For this review, use the dimensioned drawing (mm, ordinates from the lowest corner) and the shaded views. A direction names the side the tool comes from. Round coordinates to 2 decimals unless told otherwise and drop trailing zeros. Write each loop counter-clockwise with the first axis right and the second up, starting at its lowest first coordinate (ties: lowest second). Pieces come first, ordered by that corner, then holes. Notation, with made-up numbers: M 39.5,52 L 55.5,52 A18 cw 55.5,65 Z; hole C -35.5,-16.75 d10. An arc over 180 degrees is marked long. Write each question's results on one line, items separated by ' | '. Start each with the question number.
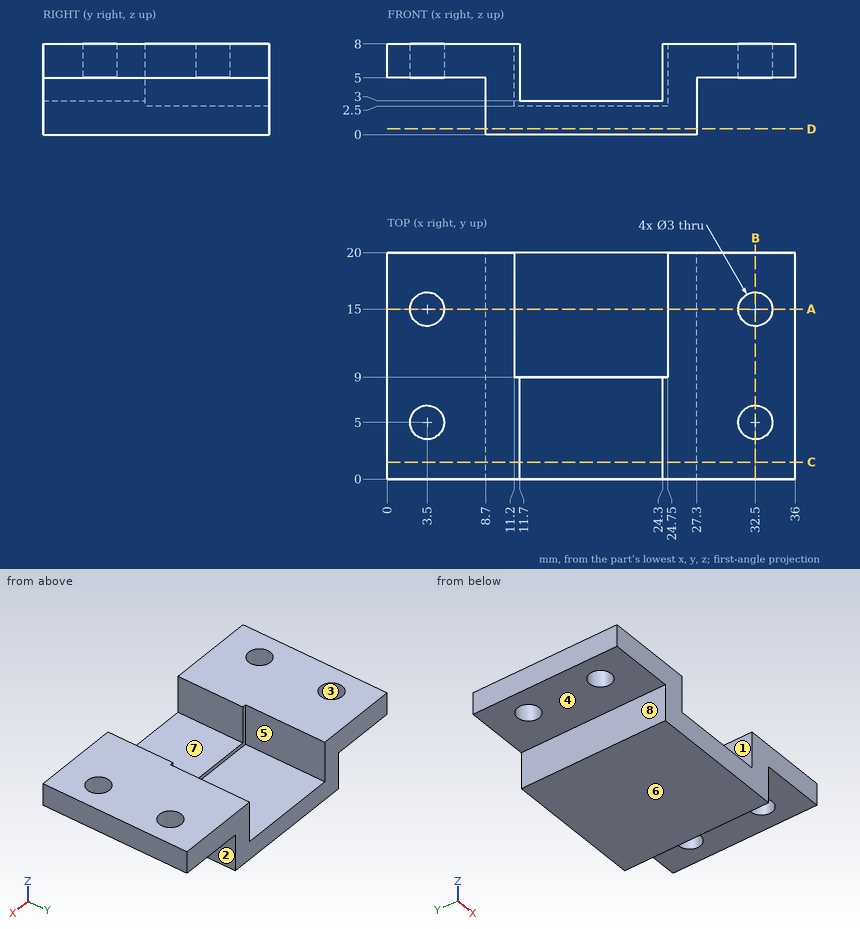
Item 1: Insertion check: P1, Ø3.5, axis at x = 15.5, y = 13, coming from the +Z side; P2, Ø7, axis at x = 19.5, y = 3.5, coming from the +Z side; P3, Ø2.5, axis at x = 3, y = 13, coming from the -Z side. Each pin has a flat end and moves straight along its axis. Give the tip position at first contact, or say it passes through.
Item 2: We need section C-C on y = 1.5. State the section outline as (x, z) points.
Item 3: For probe 1 along Y at (x, z) = (32.5, 6.95); probe 2 along X at (y, z) = (11.75, 3.25); probe 3 along X at (y, z) = (15.25, 6), list the stretches that pass through material, from the lowest coordinate up.
Item 4: We need section B-B on x = 32.5. State the section outline as (y, z) points.
Item 5: Mouldability with a two-part tool opening along X and no side actions: class the marked faces 6, 7 and 8 as pulls with the +X half, pulls with the -X half, needs draft (parallel to the pull), parting line crosses it, or undercut.
Item 6: For the marked faces 1, 2, 3, 4 and 5, list the 3-axis set-ups (+Z, -Z, +X, -X, +Y, -Y) from which the entire face can be reached by the end or side of a thin tool; tool diameter is ignored.
Item 7: We need section A-A on y = 15. State the section outline as (x, z) points, then the cut area to 3 significant figures.
Item 8: We need section D-D on z = 0.5. State the section outline as (x, y) points, then the cut area to 3 significant figures.
Numbers:
1) P1: stops at z = 2.5 | P2: stops at z = 3 | P3: stops at z = 5
2) outline: M 0,5 L 8.7,5 L 8.7,0 L 27.3,0 L 27.3,5 L 36,5 L 36,8 L 24.3,8 L 24.3,3 L 11.7,3 L 11.7,8 L 0,8 Z
3) probe 1: y = 0 to 3.5, 6.5 to 13.5, 16.5 to 20 | probe 2: x = 8.7 to 11.2, 24.75 to 27.3 | probe 3: x = 0 to 2.02, 4.98 to 11.2, 24.75 to 31.02, 33.98 to 36
4) outline: M 0,5 L 3.5,5 L 3.5,8 L 0,8 Z; M 6.5,5 L 13.5,5 L 13.5,8 L 6.5,8 Z; M 16.5,5 L 20,5 L 20,8 L 16.5,8 Z
5) face 6: needs draft | face 7: undercut | face 8: pulls with the -X half
6) face 1: +Z, +Y, -Y | face 2: -Z, +X, +Y, -Y | face 3: +Z, -Z | face 4: -Z, -X, +Y, -Y | face 5: +Z, +Y
7) outline: M 0,5 L 2,5 L 2,8 L 0,8 Z; M 5,5 L 8.7,5 L 8.7,0 L 27.3,0 L 27.3,5 L 31,5 L 31,8 L 24.75,8 L 24.75,2.5 L 11.2,2.5 L 11.2,8 L 5,8 Z; M 34,5 L 36,5 L 36,8 L 34,8 Z | area: 108 mm^2
8) outline: M 8.7,0 L 27.3,0 L 27.3,20 L 8.7,20 Z | area: 372 mm^2
